```python
from build123d import *

# Parameters (mm, degrees)
BRIDA_BASE1_DEPTH     = 7
CORTAR_EXTRUIR1_REACH = 37.355
CROQUIS6_R            = 2
CORTAR_EXTRUIR2_REACH = 37.355
CROQUIS9_R            = 2


# Sheet-metal steps are written as plain solids
with BuildPart() as part:
    # Croquis1 → Brida base1 (new, symmetric)
    with BuildSketch(Plane(origin=(0, 0, 0), x_dir=(0, 0, -1), z_dir=(1, 0, 0))):
        with BuildLine():
            Line((0, 25), (0, 1.7366))
            ThreePointArc((0, 1.7366), (-0.508638364, 0.508638364), (-1.7366, 0))
            Line((-1.7366, 0), (-25, 0))
            Line((-25, 0), (-25, 1))
            Line((-25, 1), (-1.7366, 1))
            ThreePointArc((-1.7366, 1), (-1.215745145, 1.215745145), (-1, 1.7366))
            Line((-1, 1.7366), (-1, 25))
            Line((-1, 25), (0, 25))
        make_face()
    extrude(amount=BRIDA_BASE1_DEPTH, both=True)

    # Croquis6 → Cortar-Extruir1 (cut, up to next)
    with BuildSketch(Plane.XY.offset(1), mode=Mode.PRIVATE) as cortar_extruir1_sk1:
        with Locations((0, 13)):
            Circle(CROQUIS6_R)
    cortar_extruir1_tool1 = extrude(cortar_extruir1_sk1.sketch, amount=-CORTAR_EXTRUIR1_REACH, mode=Mode.PRIVATE) & part.part
    add(cortar_extruir1_tool1.solids().sort_by_distance((0, 13, 1))[0], mode=Mode.SUBTRACT)

    # Croquis9 → Cortar-Extruir2 (cut, up to next)
    with BuildSketch(Plane(origin=(0, 1, 0), x_dir=(1, 0, 0), z_dir=(0, 1, 0)), mode=Mode.PRIVATE) as cortar_extruir2_sk1:
        with Locations(Location((0, -13, 0), (0, 0, 270))):
            Circle(CROQUIS9_R)
    cortar_extruir2_tool1 = extrude(cortar_extruir2_sk1.sketch, amount=-CORTAR_EXTRUIR2_REACH, mode=Mode.PRIVATE) & part.part
    add(cortar_extruir2_tool1.solids().sort_by_distance((0, 1, 13))[0], mode=Mode.SUBTRACT)


solid = part.part
```
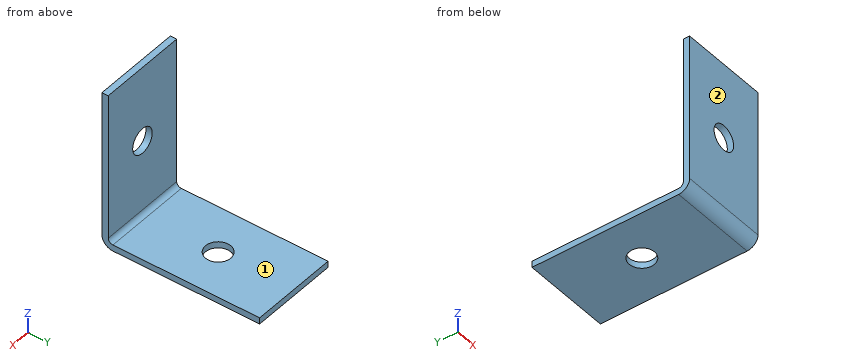
CAD build for the part. Positions are in the model's coordinates, mm. Face numbers are marked on the shaded views. A direction names the side the tool comes from. Round coordinates to 2 decimals unless told otherwise and drop trailing zeros. Order: outer loops, then holes, each group sorted by start corner. A loop starts at its lowest first (then second) coordinate and runs counter-clockwise, first axis right, second up. Notation, with made-up numbers: (-29, -38) -> (-13, -38) arc R21 ccw to (-13, -19) -> close; hole circle Ø10 at (-25, -32.5). An arc over 180 degrees is marked (long way). One line per question, with ' | ' between items.
Q1. Slice it at B-B (x = 0). Write the cut outline in (y, z), then the cut area to 3 significant figures.
Completed:
outline: (0, 1.74) arc R1.74 ccw to (1.74, 0) -> (11, 0) -> (11, 1) -> (1.74, 1) arc R0.74 cw to (1, 1.74) -> (1, 11) -> (0, 11) -> close; (0, 15) -> (1, 15) -> (1, 25) -> (0, 25) -> close; (15, 0) -> (25, 0) -> (25, 1) -> (15, 1) -> close | area: 40.5 mm^2
Q2. Slice it at D-D (z = 18). Write the cut outline in (x, y).
Completed:
outline: (-7, 0) -> (7, 0) -> (7, 1) -> (-7, 1) -> close
Q3. Probe probe 1 along X at (y, z) = (0.6, 13); probe 2 along Z at (x, y) = (-5.25, 8.25). List the from-to ranges inside material, lowest first.
Completed:
probe 1: x = -7 to -2, 2 to 7 | probe 2: z = 0 to 1
Q4. Slice it at A-A (z = 13). Write the cut outline in (x, y).
Completed:
outline: (-7, 0) -> (-2, 0) -> (-2, 1) -> (-7, 1) -> close; (2, 0) -> (7, 0) -> (7, 1) -> (2, 1) -> close
Q5. Drop flat-ended pins along their axis: pin 1 (3.5 mm diameter, centred on x = 0, z = 13, fed in from +Y); pin 2 (1.5 mm diameter, centred on x = -2, y = 8, fed in from +Z); pin 3 (5 mm diameter, centred on x = 2.5, z = 7, fed in from +Y); pin 4 (5 mm diameter, centred on x = 0, y = 13, fed in from -Z). Give the stop position or say it passes through.
Completed:
pin 1: passes through | pin 2: stops at z = 1 | pin 3: stops at y = 1 | pin 4: stops at z = 0
Q6. Which spindle directions (+Z, -Z, +X, -X, +Y, -Y) get a long thin tool onto all of the face, cutting with end or side? Do the marked faces 1 and 2. Say none if no direction does.
Completed:
face 1: +Z, +X, -X, +Y | face 2: +Z, -Z, +X, -X, -Y
